```python
from build123d import *

# Parameters (mm, degrees)
BOSS_EXTRUDE1_DEPTH = 3
FILLET1_R           = 20
CUT_EXTRUDE1_DEPTH  = 51.092414595
SKETCH3_R           = 2.6
CUT_EXTRUDE2_DEPTH  = 51.092414595
FILLET2_R           = 10
FILLET3_R           = 2


with BuildPart() as part:
    # Sketch1 → Boss-Extrude1 (new body)
    with BuildSketch(Plane.XY):
        Polygon((0, 0), (-32.5, 0), (-32.5, 38), (-24.5, 38), (-24.5, 8), (0, 8), (24.5, 8), (24.5, 38), (32.5, 38), (32.5, 0), align=None)
    extrude(amount=BOSS_EXTRUDE1_DEPTH)

    # Fillet1
    fillet1_edges = [part.edges().sort_by_distance(p)[0] for p in [
        (24.5, 8, 1.5),
        (-24.5, 8, 1.5),
    ]]
    fillet(fillet1_edges, radius=FILLET1_R)

    # Sketch2 → Cut-Extrude1 (cut, through all)
    with BuildSketch(Plane.XY.offset(3)):
        with BuildLine():
            Line((-30, 10.9), (-26.9, 10.9))
            ThreePointArc((-26.9, 10.9), (-26.1, 11.7), (-26.9, 12.5))
            Line((-26.9, 12.5), (-26.9, 29.3))
            ThreePointArc((-26.9, 29.3), (-26.1, 30.1), (-26.9, 30.9))
            Line((-26.9, 30.9), (-30, 30.9))
            ThreePointArc((-30, 30.9), (-30.8, 30.1), (-30, 29.3))
            Line((-30, 29.3), (-30, 12.5))
            ThreePointArc((-30, 12.5), (-30.8, 11.7), (-30, 10.9))
        make_face()
        with BuildLine():
            Line((26.9, 12.5), (26.9, 29.3))
            ThreePointArc((26.9, 29.3), (26.1, 30.1), (26.9, 30.9))
            Line((26.9, 30.9), (30, 30.9))
            ThreePointArc((30, 30.9), (30.8, 30.1), (30, 29.3))
            Line((30, 29.3), (30, 12.5))
            ThreePointArc((30, 12.5), (30.8, 11.7), (30, 10.9))
            Line((30, 10.9), (26.9, 10.9))
            ThreePointArc((26.9, 10.9), (26.1, 11.7), (26.9, 12.5))
        make_face()
        with BuildLine():
            Line((-15.9, 2.45), (15.9, 2.45))
            ThreePointArc((15.9, 2.45), (16.7, 1.65), (17.5, 2.45))
            Line((17.5, 2.45), (17.5, 5.55))
            ThreePointArc((17.5, 5.55), (16.7, 6.35), (15.9, 5.55))
            Line((15.9, 5.55), (-15.9, 5.55))
            ThreePointArc((-15.9, 5.55), (-16.7, 6.35), (-17.5, 5.55))
            Line((-17.5, 5.55), (-17.5, 2.45))
            ThreePointArc((-17.5, 2.45), (-16.7, 1.65), (-15.9, 2.45))
        make_face()
    extrude(amount=-CUT_EXTRUDE1_DEPTH, mode=Mode.SUBTRACT)

    # Sketch3 → Cut-Extrude2 (cut, through all)
    with BuildSketch(Plane.XY.offset(3)):
        with Locations((-21.4, 9.55)):
            Circle(SKETCH3_R)
        with Locations(Location((21.4, 9.55, 0), (0, 0, 180))):
            Circle(SKETCH3_R)
    extrude(amount=-CUT_EXTRUDE2_DEPTH, mode=Mode.SUBTRACT)

    # Fillet2
    fillet2_edges = [part.edges().sort_by_distance(p)[0] for p in [
        (32.5, 0, 1.5),
        (-32.5, 0, 1.5),
    ]]
    fillet(fillet2_edges, radius=FILLET2_R)

    # Fillet3
    fillet3_edges = [part.edges().sort_by_distance(p)[0] for p in [
        (24.5, 38, 1.5),
        (32.5, 38, 1.5),
        (-32.5, 38, 1.5),
        (-24.5, 38, 1.5),
    ]]
    fillet(fillet3_edges, radius=FILLET3_R)


solid = part.part
```
The model under review builds one solid part; all positions refer to its coordinate system, in mm. A direction names the side the tool comes from. Round coordinates to 2 decimals unless told otherwise and drop trailing zeros. Loops run counter-clockwise (first coordinate to the right, second up) from the corner with the lowest first, then second, coordinate; pieces in that order, holes last. Notation, with made-up numbers: M 45.5,63 L 67.5,63 A15 cw 67.5,70 Z; hole C 52,81.5 d2. An arc over 180 degrees is marked long. Put each result on its own line as item: value.
Q1. Consider section D-D, the plane z = 2.15. Count the separate pieces of the cut face and the enclosed holes in it, then the cut area to 3 significant figures.
Result set:
separate pieces: 1
enclosed holes: 5
area: 838 mm²
Q2. For pin 1 (0.9 mm diameter, centred on y = 4, z = 2, fed in from +X); pin 2 (0.9 mm diameter, centred on y = 3.5, z = 1, fed in from -X); pin 3 (1.5 mm diameter, centred on x = 0, z = 2, fed in from +Y), all flat-tipped, find the tip position at first contact; note any pin that passes through.
Result set:
pin 1: stops at x = 30.82
pin 2: stops at x = -30.46
pin 3: stops at y = 8
Q3. Machinability: for faces 4 (the flat face through (-24.5, 32, 1)), 5 (the cylindrical face through (31.93, 37.4, 1.52)), 6 (the cylindrical face through (30.8, 30.1, 1.5)), which of the approach directions +Z, -Z, +X, -X, +Y, -Y give a long, thin tool a straight path to every point of the face, cutting with its end or side? Answer none if there is none.
Result set:
face 4: +Z, -Z, +Y
face 5: +Z, -Z, +X, +Y
face 6: +Z, -Z
Q4. To check wall thickness, follow L1, parallel to X at y = 28.5, z = 1.3; L2, parallel to Y at x = 4, z = 2.55; L3, parallel to X at y = 25, z = 1.4. State the ranges of each line that lie inside material, in increasing order.
Result set:
L1: x = -32.5 to -30, -26.9 to -24.5, 24.5 to 26.9, 30 to 32.5
L2: y = 0 to 2.45, 5.55 to 8
L3: x = -32.5 to -30, -26.9 to -24.27, 24.27 to 26.9, 30 to 32.5
Q5. Consider section B-B, the plane y = 32. Give the boundary of the cut face in (x, z), then the cut area to 3 significant figures.
Result set:
outline: M -32.5,0 L -24.5,0 L -24.5,3 L -32.5,3 Z; M 24.5,0 L 32.5,0 L 32.5,3 L 24.5,3 Z
area: 48.0 mm²
Q6. Consider section A-A, the plane x = -1. Give the boundary of the cut face in (y, z).
Result set:
outline: M 0,0 L 2.45,0 L 2.45,3 L 0,3 Z; M 5.55,0 L 8,0 L 8,3 L 5.55,3 Z
Q7. Consider section C-C, the plane y = 26. Give the boundary of the cut face in (x, z).
Result set:
outline: M -32.5,0 L -30,0 L -30,3 L -32.5,3 Z; M -26.9,0 L -24.4,0 L -24.4,3 L -26.9,3 Z; M 24.4,0 L 26.9,0 L 26.9,3 L 24.4,3 Z; M 30,0 L 32.5,0 L 32.5,3 L 30,3 Z
Q8. Mouldability with a two-part tool opening along X and no side actions: class faces 1 (the flat face through (30, 21, 2)), 2 (the flat face through (-29, 38, 1)), 3 (the cylindrical face through (-29.65, 3.01, 1.52)) as released by +X, released by -X, zero draft, split by the parting line, or undercut.
Result set:
face 1: undercut
face 2: zero draft
face 3: released by -X
